Job drawing, mm, ordinate dimensions from the low corner. One solid piece. A direction names the side the tool comes from. Give positions to 0.01 mm unless a question says otherwise; leave off trailing zeros. Loops run counter-clockwise (first coordinate to the right, second up) from the corner with the lowest first, then second, coordinate; pieces in that order, holes last.
Item 1: Saw through at A-A on x = 3. Give the cut face in (y, z).
Item 2: Which spindle directions (+Z, -Z, +X, -X, +Y, -Y) get a long thin tool onto all of the face, cutting with end or side? Do the marked faces 1 and 2. Say none if no direction does.
Item 3: Drop a flat-ended pin along its axis: P1, Ø1, axis at y = 1, z = 2, coming from the -X side. Give the stop position or say it passes through.
Item 4: Saw through at C-C on z = 1.25. Give the cut face in (x, y).
Item 5: Probe probe 1 along Y at (x, z) = (3, 5); probe 2 along Y at (x, z) = (2.1, 5); probe 3 along X at (y, z) = (2.75, 5.25). List the from-to ranges inside material, lowest first.
Item 6: Mould opens along Y. For the marked faces 3, 4 and 5 say: released by +Y, released by -Y, zero draft, split by the parting line, or undercut.
Item 7: Saw through at D-D on x = 1.3. Give the cut face in (y, z), plus the area to 3 significant figures.
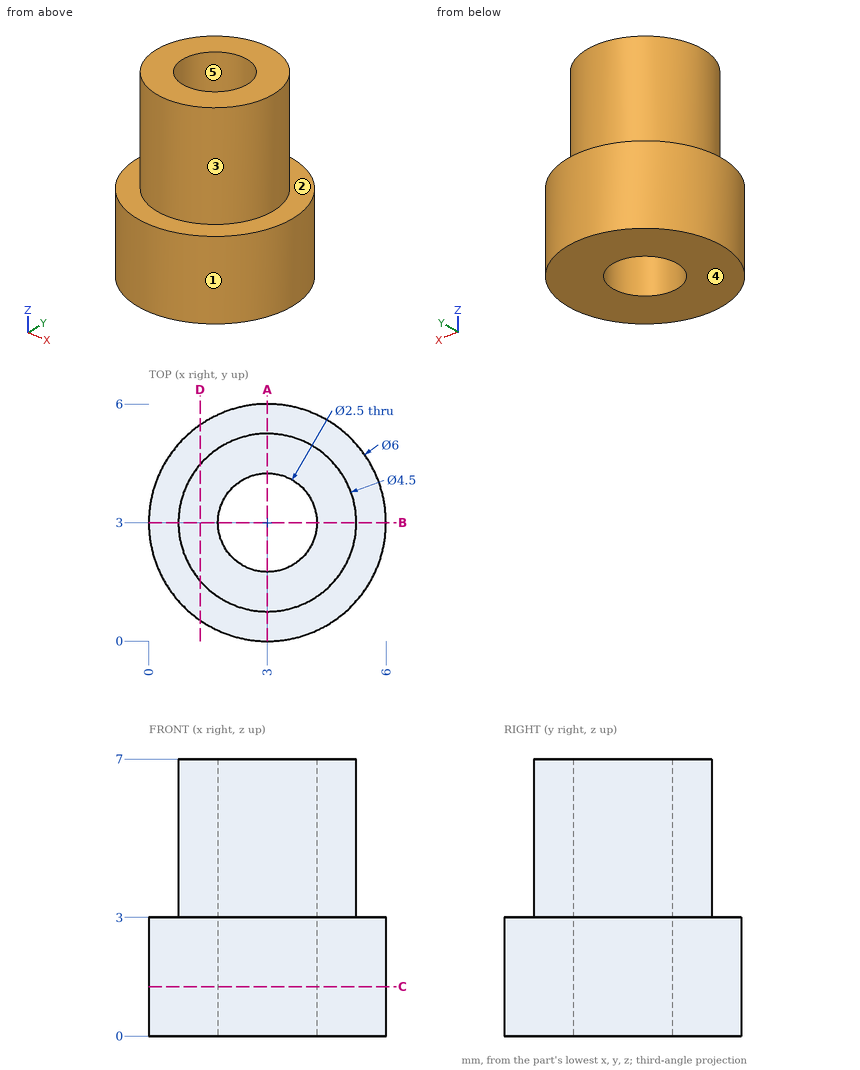
Results below:
1. outline: (0, 0) - (1.75, 0) - (1.75, 7) - (0.75, 7) - (0.75, 3) - (0, 3) - close; (4.25, 0) - (6, 0) - (6, 3) - (5.25, 3) - (5.25, 7) - (4.25, 7) - close
2. face 1: +Z, -Z
2. face 2: +Z
3. P1: stops at x = 0.4
4. outline: circle Ø6 at (3, 3); hole circle Ø2.5 at (3, 3)
5. probe 1: y = 0.75 to 1.75, 4.25 to 5.25
5. probe 2: y = 0.94 to 2.13, 3.87 to 5.06
5. probe 3: x = 0.76 to 1.78, 4.22 to 5.24
6. face 3: split by the parting line
6. face 4: zero draft
6. face 5: undercut
7. outline: (0.53, 0) - (5.47, 0) - (5.47, 3) - (4.47, 3) - (4.47, 7) - (1.53, 7) - (1.53, 3) - (0.53, 3) - close
7. area: 26.6 mm2
